from build123d import *

# Parameters (mm, degrees)
EXTRUDE_1_DEPTH     = 10
FILLET_2_R          = 3
SKETCH_2_R          = 1.5
CUT_EXTRUDE_1_DEPTH = 7


with BuildPart() as part:
    # 草图1 → 凸台-拉伸1 (new body)
    with BuildSketch(Plane(origin=(0, 0, 0), x_dir=(1, 0, 0), z_dir=(0, 1, 0))):
        with BuildLine():
            Line((35.177708011, -0.253238784), (35.667337743, -0.253238784))
            ThreePointArc((35.667337743, -0.253238784), (36.384198182, 0.049544528), (36.666951866, 0.774538994))
            ThreePointArc((36.666951866, 0.774538994), (-0.318770688, 36.746761216), (-37.304493242, 0.774538994))
            ThreePointArc((-37.304493242, 0.774538994), (-37.021739558, 0.049544528), (-36.304879119, -0.253238784))
            Line((-36.304879119, -0.253238784), (-35.815249387, -0.253238784))
            Line((-35.815249387, -0.253238784), (-34.959786839, -0.253238784))
            ThreePointArc((-34.959786839, -0.253238784), (-0.330707465, 29.746759181), (34.318826897, -0.229611257))
            Line((34.318826897, -0.229611257), (35.177708011, -0.253238784))
        make_face()
    extrude(amount=EXTRUDE_1_DEPTH)

    # 圆角2
    fillet_2_edges = [part.edges().sort_by_distance(p)[0] for p in [
        (-0.330707465, 10, -29.746759181),
    ]]
    fillet(fillet_2_edges, radius=FILLET_2_R)

    # 草图2 → 切除-拉伸1 (cut)
    with BuildSketch(Plane.XZ):
        with Locations(Location((-15.318770688, -29.700892818, 0), (0, 0, 270))):
            Circle(SKETCH_2_R)
        with Locations(Location((14.681229312, -29.700892818, 0), (0, 0, 90))):
            Circle(SKETCH_2_R)
    extrude(amount=-CUT_EXTRUDE_1_DEPTH, mode=Mode.SUBTRACT)


solid = part.part
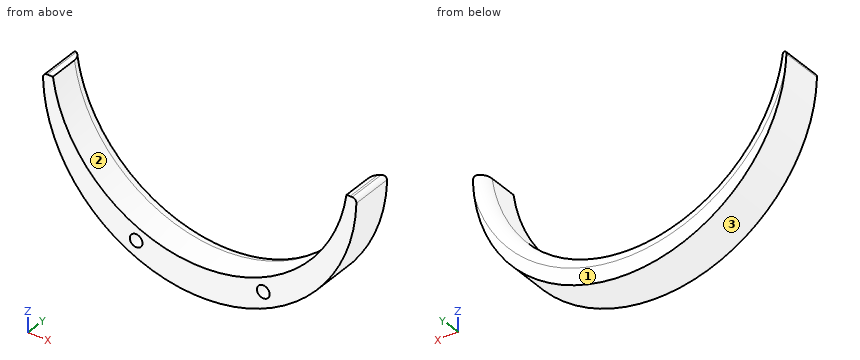
Can you work these out from the model? Positions are in its coordinate system, mm. Face numbers are marked on the shaded views. Coordinates: 2 decimals unless noted, no trailing zeros. Write each loop counter-clockwise with the first axis right and the second up, starting at its lowest first coordinate (ties: lowest second). Pieces come first, ordered by that corner, then holes. Notation, with made-up numbers: (87, 24) - (108, 24) arc R34 cw to (108, 62) - close; hole circle Ø10 at (87, 43). An arc over 180 degrees is marked (long way). Return JSON: item names as keys, results as strings. Group by question number.
Item 1: I'm going to push flat-ended pins straight in: pin 1 Ø4 at (x, y) = (-10, 3) entering from -Z; pin 2 Ø2.5 at (x, z) = (15, -29) entering from -Y; pin 3 Ø2 at (x, z) = (-27.5, -26.5) entering from +Y; pin 4 Ø2 at (y, z) = (5.5, -13) entering from +X. Where does each tip first touch, or does it pass through?
Item 2: Please list where these lines run through material, in increasing order: probe 1 along X at (y, z) = (3.5, -24); probe 2 along Z at (x, y) = (14, 4); probe 3 along X at (y, z) = (7.5, -17).
Item 3: We'd pull the mould along X, two halves only. Please class the marked faces 1, 2 and 3: pulls with the +X half, pulls with the -X half, needs draft (parallel to the pull), parting line crosses it, or undercut.
Item 4: If we section it at A-A (y = 5.5): Write out the boundary of the cut face in (x, z).
Return value:
{
 "1": {"pin 1": "stops at z = -35.94", "pin 2": "stops at y = 0", "pin 3": "passes through", "pin 4": "stops at x = 34.59"},
 "2": {"probe 1": "x = -28.26 to -19.53, 18.9 to 27.62", "probe 2": "z = -33.86 to -31.04, -28.36 to -26.68", "probe 3": "x = -33.05 to -27.39, 26.75 to 32.41"},
 "3": {"face 1": "needs draft", "face 2": "undercut", "face 3": "parting line crosses it"},
 "4": {"outline": "(-37.3, -0.77) arc R37 ccw to (36.67, -0.77) arc R1 ccw to (35.67, 0.25) - (35.18, 0.25) - (34.32, 0.23) arc R35 cw to (-34.96, 0.25) - (-36.3, 0.25) arc R1 ccw to start; hole circle Ø3 at (-15.32, -29.7); hole circle Ø3 at (14.68, -29.7)"}
}
